```python
from build123d import *

# Parameters (mm, degrees)
F0_W      = 16
F0_H      = 16
F1_DEPTH  = 8
F2_R      = 2
F3_R      = 1.75
F4_DEPTH  = 1
F5_R      = 1.75
F6_DEPTH  = 1
F7_R      = 1.75
F8_DEPTH  = 1
F9_R      = 1.75
F10_DEPTH = 1
F11_R     = 1.75
F12_DEPTH = 1
F13_R     = 1.75
F14_DEPTH = 1


with BuildPart() as f1:
    # F0 (on Front) → F1 (new body, symmetric)
    with BuildSketch(Plane.XZ):
        Rectangle(F0_W, F0_H)
    extrude(amount=F1_DEPTH, both=True)

    # F2
    f2_edges = [f1.edges().sort_by_distance(p)[0] for p in [
        (0, -8, 8),
        (8, 0, 8),
        (8, -8, 0),
        (8, 8, 0),
        (8, 0, -8),
        (0, -8, -8),
        (0, 8, -8),
        (0, 8, 8),
        (-8, 8, 0),
        (-8, -8, 0),
        (-8, 0, -8),
        (-8, 0, 8),
    ]]
    fillet(f2_edges, radius=F2_R)

    # F3 (on face) → F4 (cut)
    with BuildSketch(Plane(origin=(-8, 0, 0), x_dir=(0, -1, 0), z_dir=(-1, 0, 0))):
        Circle(F3_R)
    extrude(amount=-F4_DEPTH, mode=Mode.SUBTRACT)

    # F5 (on face) → F6 (cut)
    with BuildSketch(Plane.XZ.offset(8)):
        with Locations((3.193169, 3.366647)):
            Circle(F5_R)
        with Locations((-3.031091, -3.203825)):
            Circle(F5_R)
    extrude(amount=-F6_DEPTH, mode=Mode.SUBTRACT)

    # F7 (on face) → F8 (cut)
    with BuildSketch(Plane.YZ.offset(8)):
        with Locations((-3.87646, 3.926625)):
            Circle(F7_R)
        with Locations((-3.87646, 0)):
            Circle(F7_R)
        with Locations((-3.87646, -4.054355)):
            Circle(F7_R)
        with Locations((4.099085, 3.926625)):
            Circle(F7_R)
        with Locations((4.099085, 0)):
            Circle(F7_R)
        with Locations((4.099085, -4.054355)):
            Circle(F7_R)
    extrude(amount=-F8_DEPTH, mode=Mode.SUBTRACT)

    # F9 (on face) → F10 (cut)
    with BuildSketch(Plane(origin=(0, 8, 0), x_dir=(-1, 0, 0), z_dir=(0, 1, 0))):
        Circle(F9_R)
        with Locations((3.661382, 4.083229)):
            Circle(F9_R)
        with Locations((-3.603264, 4.083229)):
            Circle(F9_R)
        with Locations((-3.603264, -3.550806)):
            Circle(F9_R)
        with Locations((3.661382, -3.550806)):
            Circle(F9_R)
    extrude(amount=-F10_DEPTH, mode=Mode.SUBTRACT)

    # F11 (on face) → F12 (cut)
    with BuildSketch(Plane.XY.offset(8)):
        Circle(F11_R)
        with Locations((3.39505, -3.466212)):
            Circle(F11_R)
        with Locations((-3.431327, 3.261353)):
            Circle(F11_R)
    extrude(amount=-F12_DEPTH, mode=Mode.SUBTRACT)

    # F13 (on face) → F14 (cut)
    with BuildSketch(Plane(origin=(0, 0, -8), x_dir=(1, 0, 0), z_dir=(0, 0, -1))):
        with Locations((-3.193001, 2.974751)):
            Circle(F13_R)
        with Locations((3.554628, 2.974751)):
            Circle(F13_R)
        with Locations((3.554628, -2.995252)):
            Circle(F13_R)
        with Locations((-3.193001, -2.995252)):
            Circle(F13_R)
    extrude(amount=-F14_DEPTH, mode=Mode.SUBTRACT)


solid = f1.part
```
Can you work these out from the model? Positions are in its coordinate system, mm. A direction names the side the tool comes from. Give positions to 0.01 mm unless a question says otherwise; leave off trailing zeros. Order: outer loops, then holes, each group sorted by start corner. A loop starts at its lowest first (then second) coordinate and runs counter-clockwise, first axis right, second up. Notation, with made-up numbers: M -11.75,15 L 43.25,15 A9 cw 43.25,28 Z; hole C 51,55 d7. An arc over 180 degrees is marked long. Write item = value, one per line. Start each with the question number.
Q1. Suppose I cut it at C-C (z = 0). Write out the boundary of the cut face in (x, y), plus the area to 3 significant figures.
Q2. Suppose I cut it at A-A (y = 0). Write out the boundary of the cut face in (x, z), plus the area to 3 significant figures.
Q3. For faces 1 (the flat face through (0, 0, 7)), 2 (the cylindrical face through (5.17, 3.67, -7.51)), 3 (the cylindrical face through (7.507, -3.069, 2.374)), which set-ups out of +Z, -Z, +X, -X, +Y, -Y let a thin tool reach every point of the face, with its end or its side?
Q4. Will these pins go through, and if not, where does the flat tip stop? pin 1 Ø3 at (x, z) = (0, 0) entering from +Y; pin 2 Ø1 at (x, z) = (3, 4) entering from -Y; pin 3 Ø1 at (x, y) = (3, -4) entering from +Z.
Q5. Suppose I cut it at B-B (x = 0). Write out the boundary of the cut face in (y, z).
Q6. I need wall thicknesses on probe 1 along Z at (x, y) = (-3.5, 1.75); probe 2 along Z at (x, y) = (4, 1.5). Which ranges of each line are inside material? Lowest first, please. Write a range as [from, to].
Q7. We'd pull the mould along Y, two halves only. Please class faces 4 (the flat face through (3, -7, 3)), 5 (the cylindrical face through (7.43, -0.08, -7.4)), 6 (the flat face through (7, -4, -4)): pulls with the +Y half, pulls with the -Y half, needs draft (parallel to the pull), parting line crosses it, or undercut.
Check result:
q1.outline = M -8,-6 A2 ccw -6,-8 L 6,-8 A2 ccw 8,-6 L 8,-5.63 L 7,-5.63 L 7,-2.13 L 8,-2.13 L 8,2.35 L 7,2.35 L 7,5.85 L 8,5.85 L 8,6 A2 ccw 6,8 L 1.75,8 L 1.75,7 L -1.75,7 L -1.75,8 L -6,8 A2 ccw -8,6 L -8,1.75 L -7,1.75 L -7,-1.75 L -8,-1.75 Z
q1.area = 239 mm2
q2.outline = M -8,-6 A2 ccw -6,-8 L 6,-8 A2 ccw 8,-6 L 8,6 A2 ccw 6,8 L 1.75,8 L 1.75,7 L -1.75,7 L -1.75,8 L -6,8 A2 ccw -8,6 L -8,1.75 L -7,1.75 L -7,-1.75 L -8,-1.75 Z
q2.area = 246 mm2
q3.face_1 = +Z
q3.face_2 = -Z
q3.face_3 = +X
q4.pin_1 = 7
q4.pin_2 = -7
q4.pin_3 = 7
q5.outline = M -8,-6 A2 ccw -6,-8 L 6,-8 A2 ccw 8,-6 L 8,-1.75 L 7,-1.75 L 7,1.75 L 8,1.75 L 8,6 A2 ccw 6,8 L 1.75,8 L 1.75,7 L -1.75,7 L -1.75,8 L -6,8 A2 ccw -8,6 Z
q6.probe_1 = [-7, 7]
q6.probe_2 = [-7, 8]
q7.face_4 = pulls with the -Y half
q7.face_5 = needs draft
q7.face_6 = undercut
